```python
from build123d import *

# Parameters (mm, degrees)
FILLET1_R           = 2.5
SKETCH2_R           = 2.443196487
BOSS_EXTRUDE1_DEPTH = 15


with BuildPart() as part:
    # Sketch1 → Revolve1 (revolve)
    with BuildSketch(Plane.XY, mode=Mode.PRIVATE) as revolve1_sk:
        Polygon((0, 0), (0, 110), (2.5, 110), (5, 0), align=None)
    revolve(revolve1_sk.sketch.rotate(Axis((0, 0, 0), (0, 1, 0)), 90), axis=Axis((0, 0, 0), (0, 1, 0)))

    # Fillet1
    fillet1_edges = [part.edges().sort_by_distance(p)[0] for p in [
        (0, 110, 2.5),
        (0, 0, 5),
    ]]
    fillet(fillet1_edges, radius=FILLET1_R)

    # Sketch2 → Boss-Extrude1 (add)
    with BuildSketch(Plane(origin=(0, 0, 0), x_dir=(0, 0, -1), z_dir=(1, 0, 0))):
        with Locations(Location((0, 5, 0), (0, 0, 269.999999999))):
            Circle(SKETCH2_R)
    extrude(amount=BOSS_EXTRUDE1_DEPTH)


solid = part.part
```
Work out the finished part from the listing and answer in its coordinate system (mm). A direction names the side the tool comes from. Give positions to 0.01 mm unless a question says otherwise; leave off trailing zeros. Loops run counter-clockwise (first coordinate to the right, second up) from the corner with the lowest first, then second, coordinate; pieces in that order, holes last. Notation, with made-up numbers: (80.5, 39) -> (129.5, 39) arc R26 ccw to (129.5, 74) -> close; hole circle Ø1 at (-6, 8.5). An arc over 180 degrees is marked (long way). Put each result on its own line as item: value. Start each with the question number.
Item 1: Each of these flat-tipped pins is pushed along its axis until it touches: P1, Ø3, axis at x = 11.5, z = 2, coming from the +Y side; P2, Ø5, axis at x = 5.5, z = 1.5, coming from the -Y side; P3, Ø3, axis at x = -1.5, y = 11.5, coming from the +Z side. Where does it stop, or does it pass through?
Item 2: Which of the six approach directions +Z, -Z, +X, -X, +Y, -Y give full straight-line access (tool end or side, diameter ignored) to faces 1 (the face through (0, 0, 0)), 2 (the face through (9.54, 7.44, -0.11))?
Item 3: The part is cut by section A-A (y = 22). Give the vertices of the cut face in (x, z), then the cut area to 3 significant figures.
Item 4: The part is cut by section B-B (y = 99). Give the vertices of the cut face in (x, z).
Item 5: Find the intervals of material crossed by L1, parallel to X at y = 94.5, z = -0.25; L2, parallel to Y at x = 1, z = -1.75; L3, parallel to Z at x = -1.25, y = 80.5, in increasing order. Write a range as [from, to].
Item 6: The part is cut by section C-C (y = 5). Give the vertices of the cut face in (x, z), then the cut area to 3 significant figures.
Item 7: The mould has two halves that part along Z. Classify faces 3 (the face through (2.29, 54.32, 2.99)), 4 (the face through (15, 5, 0)): released by +Z, released by -Z, zero draft, split by the parting line, or undercut.
Answers below:
1. P1: y = 7.39
1. P2: y = 0.12
1. P3: z = 4.75
2. face 1: +Z, -Z, +X, -X, -Y
2. face 2: +X
3. outline: circle Ø9 at (0, 0)
3. area: 63.6 mm2
4. outline: circle Ø5.5 at (0, 0)
5. L1: [-2.84, 2.84]
5. L2: [0, 109.05]
5. L3: [-2.91, 2.91]
6. outline: (4.23, -2.44) -> (15, -2.44) -> (15, 2.44) -> (4.23, 2.44) arc R4.89 ccw (long way) to start
6. area: 125 mm2
7. face 3: split by the parting line
7. face 4: zero draft
